```python
from build123d import *

# Parameters (mm, degrees)
F2_R     = 8.877564
F3_DEPTH = 98.5
F4_R     = 9.157868
F5_DEPTH = 80.2
F7_DEPTH = 93.5


with BuildPart() as f1:
    # F0 (on Front) → F1 (revolve)
    with BuildSketch(Plane.XZ):
        with BuildLine():
            Line((0, 59.798335), (0, -59.798335))
            ThreePointArc((0, -59.798335), (59.798335, 0), (0, 59.798335))
        make_face()
    revolve(axis=Axis((0, 0, 0), (0, 0, -1)))

    # F2 (on Front) → F3 (cut, symmetric)
    with BuildSketch(Plane.XZ):
        with Locations((-26.740938, 22.834959)):
            Circle(F2_R)
    extrude(amount=F3_DEPTH, both=True, mode=Mode.SUBTRACT)

    # F4 (on Front) → F5 (cut, symmetric)
    with BuildSketch(Plane.XZ):
        with Locations((25.83956, 23.435879)):
            Circle(F4_R)
    extrude(amount=F5_DEPTH, both=True, mode=Mode.SUBTRACT)

    # F6 (on Front) → F7 (cut, symmetric)
    with BuildSketch(Plane.XZ):
        with BuildLine():
            ThreePointArc((22.971286, -20.687239), (1.648874, -21.786302), (-19.701775, -21.840565))
            ThreePointArc((-19.701775, -21.840565), (2.043902, -36.402335), (22.971286, -20.687239))
        make_face()
    extrude(amount=F7_DEPTH, both=True, mode=Mode.SUBTRACT)


solid = f1.part
```
Design review of the part built by this model. Coordinates are the model's own, in mm. Give positions to 0.01 mm unless a question says otherwise; leave off trailing zeros. Order: outer loops, then holes, each group sorted by start corner. A loop starts at its lowest first (then second) coordinate and runs counter-clockwise, first axis right, second up. Notation, with made-up numbers: M 7,41.5 L 19,41.5 A18 cw 19,69.5 Z; hole C 2,9 d9. An arc over 180 degrees is marked long. One line per question, with ' | ' between items. Start each with the question number.
Q1. For L1, parallel to Z at x = -17.5, y = -21; L2, parallel to X at y = 30.5, z = -34.5; L3, parallel to Y at x = 19, z = 10.5, list the stretches that pass through material, from the lowest coordinate up. Write a range as [from, to].
Q2. We need section C-C (x = 8.5). Write out the cut boundary in (y, z).
Q3. For pin 1 Ø1 at (x, y) = (-23.5, -7.5) entering from +Z; pin 2 Ø1 at (x, y) = (-30.5, 12) entering from -Z; pin 3 Ø10 at (x, y) = (25, 20) entering from +Z; pin 4 Ø14.5 at (x, z) = (25.84, 23.44) entering from +Y, all flat-tipped, find the tip position at first contact; note any pin that passes through.
Q4. We need section B-B (y = -20). Write out the cut boundary in (x, z).
Q5. We need section A-A (x = 21). Write out the cut boundary in (y, z).
Q6. We need section D-D (z = 53). Write out the cut boundary in (x, y), plus the area to 3 significant figures.
Returned:
1) L1: [-53.18, -26.16], [-21.88, 53.18] | L2: [-38.15, -7.66], [10.53, 38.15] | L3: [-55.72, 55.72]
2) outline: M -55.13,-21.55 L 55.13,-21.55 A59.19 ccw long Z; M -47.53,-35.28 A59.19 ccw 47.53,-35.28 Z
3) pin 1: z = 54.7 | pin 2: z = -50.34 | pin 3: z = 53.35 | pin 4: through
4) outline: C 0,0 d112.71; hole C -26.74,22.83 d17.76; hole M -19.7,-21.84 A22.61 ccw 22.97,-20.69 A436.15 cw Z; hole C 25.84,23.44 d18.32
5) outline: M -53.75,15.66 A55.99 ccw -51.97,-20.83 L 51.97,-20.83 A55.99 ccw 53.75,15.66 Z; M -50.03,-25.13 A55.99 ccw 50.03,-25.13 Z; M -46.48,31.21 L 46.48,31.21 A55.99 ccw Z
6) outline: C 0,0 d55.38 | area: 2,410 mm2
